```python
from build123d import *

# Parameters (mm, degrees)
SKETCH1_R           = 12
BOSS_EXTRUDE1_DEPTH = 29
SKETCH2_R           = 3
BOSS_EXTRUDE2_DEPTH = 1
SKETCH3_R           = 1
BOSS_EXTRUDE3_DEPTH = 10


with BuildPart() as part:
    # Sketch1 → Boss-Extrude1 (new body)
    with BuildSketch(Plane.XY):
        with Locations(Location((0, 0, 0), (0, 0, 180))):
            Circle(SKETCH1_R)
    extrude(amount=BOSS_EXTRUDE1_DEPTH)

    # Sketch2 → Boss-Extrude2 (add)
    with BuildSketch(Plane.XY.offset(29)):
        Circle(SKETCH2_R)
    extrude(amount=BOSS_EXTRUDE2_DEPTH)

    # Sketch3 → Boss-Extrude3 (add)
    with BuildSketch(Plane.XY.offset(30)):
        Circle(SKETCH3_R)
    extrude(amount=BOSS_EXTRUDE3_DEPTH)


solid = part.part
```
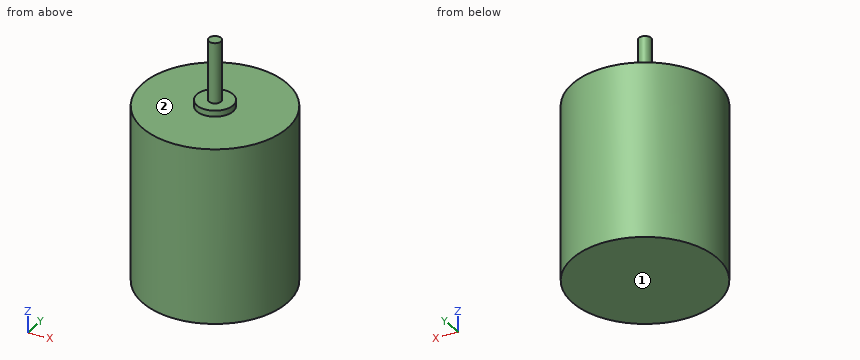
Input: part model. Units: mm. Frame: model coordinates. Face numbers are marked on the shaded views. A direction names the side the tool comes from. Coordinates: 2 decimals unless noted, no trailing zeros. Order: outer loops, then holes, each group sorted by start corner. A loop starts at its lowest first (then second) coordinate and runs counter-clockwise, first axis right, second up. Notation, with made-up numbers: (-25, 33.5) - (-9, 33.5) arc R17 cw to (-9, 46.5) - close; hole circle Ø1 at (82.5, 10). An arc over 180 degrees is marked (long way). Put each result on its own line as item: value.
1. Line query: line 1 along Z through (x, y) = (-1.5, -0.25); line 2 along Z through (x, y) = (-0.75, -7); line 3 along X through (y, z) = (-0.25, 17.5). Output: solid intervals per line, ascending.
Report:
line 1: z = 0 to 30
line 2: z = 0 to 29
line 3: x = -12 to 12
2. Reachability of the marked faces 1 and 2 from +Z, -Z, +X, -X, +Y, -Y: full face, straight path, thin tool, end or side. Return the list, or none.
Report:
face 1: -Z, +X, -X, +Y, -Y
face 2: +Z
3. Cut plane A-A on y = 0. Return the cut outline in (x, z), then the cut area to 3 significant figures.
Report:
outline: (-12, 0) - (12, 0) - (12, 29) - (3, 29) - (3, 30) - (1, 30) - (1, 40) - (-1, 40) - (-1, 30) - (-3, 30) - (-3, 29) - (-12, 29) - close
area: 722 mm2
4. Cut plane D-D on y = 2.5. Return the cut outline in (x, z).
Report:
outline: (-11.74, 0) - (11.74, 0) - (11.74, 29) - (1.66, 29) - (1.66, 30) - (-1.66, 30) - (-1.66, 29) - (-11.74, 29) - close
5. Contact query for flat-ended pins moving along their axis: pin 1 Ø2 at (y, z) = (-9, 27.5) entering from +X; pin 2 Ø3 at (x, y) = (8, -8.5) entering from +Z; pin 3 Ø5 at (y, z) = (6, 4.5) entering from -X; pin 4 Ø6.5 at (x, y) = (1, 0.5) entering from +Z. Output: stop coordinate, or through.
Report:
pin 1: stops at x = 8.94
pin 2: stops at z = 29
pin 3: stops at x = -11.48
pin 4: stops at z = 40
6. Cut plane C-C on z = 24. Return the cut outline in (x, y), then the cut area to 3 significant figures.
Report:
outline: circle Ø24 at (0, 0)
area: 452 mm2
